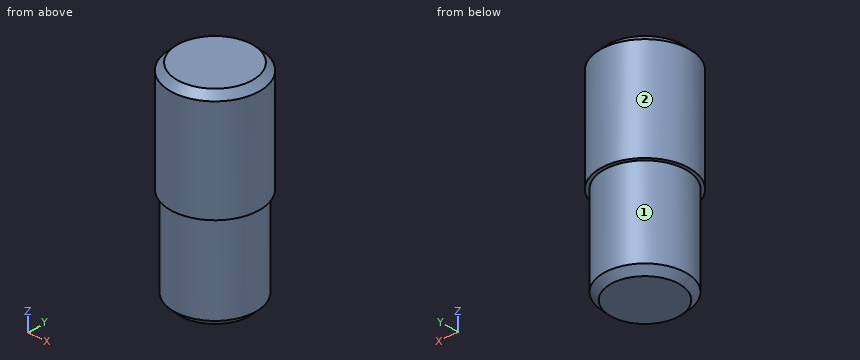
```python
from build123d import *

# Parameters (mm, degrees)
F2_SIZE = 0.5
F3_SIZE = 0.5


with BuildPart() as f1:
    # F0 (on Front) → F1 (revolve)
    with BuildSketch(Plane.XZ):
        Polygon((0, -7), (0, 0), (0, 8), (-3.25, 8), (-3.25, 0), (-3, 0), (-3, -7), align=None)
    revolve(axis=Axis((0, 0, 4), (0, 0, 1)))

    # F2
    f2_edges = [f1.edges().sort_by_distance(p)[0] for p in [
        (3.25, 0, 8),
    ]]
    chamfer(f2_edges, length=F2_SIZE)

    # F3
    f3_edges = [f1.edges().sort_by_distance(p)[0] for p in [
        (3, 0, -7),
    ]]
    chamfer(f3_edges, length=F3_SIZE)


solid = f1.part
```
CAD build for the part. Positions are in the model's coordinates, mm. Face numbers are marked on the shaded views. A direction names the side the tool comes from. Round coordinates to 2 decimals unless told otherwise and drop trailing zeros. Order: outer loops, then holes, each group sorted by start corner. A loop starts at its lowest first (then second) coordinate and runs counter-clockwise, first axis right, second up.
Q1. Drop flat-ended pins along their axis: pin 1 (2 mm diameter, centred on x = 2, z = -1.5, fed in from -Y); pin 2 (1.5 mm diameter, centred on x = 1, z = -5, fed in from -Y). Give the stop position or say it passes through.
Q2. Which spindle directions (+Z, -Z, +X, -X, +Y, -Y) get a long thin tool onto all of the face, cutting with end or side? Do the marked faces 1 and 2. Say none if no direction does.
Q3. Slice it at B-B (z = 2.25). Write the cut outline in (x, y), and give its area (3 significant figures).
Q4. Slice it at A-A (x = 0). Write the cut outline in (y, z), and give its area (3 significant figures).
Q5. Slice it at C-C (z = -6). Write the cut outline in (x, y).
Q6. Wall check: L1, parallel to X at y = 0.25, z = 6.75; L2, parallel to Z at x = -2.25, y = 2.25; L3, parallel to Y at x = 2.5, z = -2.25. Give the ranges that are in metal, low to high.
Results below:
1. pin 1: stops at y = -2.83
1. pin 2: stops at y = -2.99
2. face 1: -Z
2. face 2: +Z, -Z
3. outline: circle Ø6.5 at (0, 0)
3. area: 33.2 mm2
4. outline: (-3.25, 0) - (-3, 0) - (-3, -6.5) - (-2.5, -7) - (2.5, -7) - (3, -6.5) - (3, 0) - (3.25, 0) - (3.25, 7.5) - (2.75, 8) - (-2.75, 8) - (-3.25, 7.5) - close
4. area: 93.5 mm2
5. outline: circle Ø6 at (0, 0)
6. L1: x = -3.24 to 3.24
6. L2: z = 0 to 7.57
6. L3: y = -1.66 to 1.66
